Input: part model. Units: mm. Frame: model coordinates. Coordinates: 2 decimals unless noted, no trailing zeros. One line per question, with ' | ' between items. Start each with the question number.
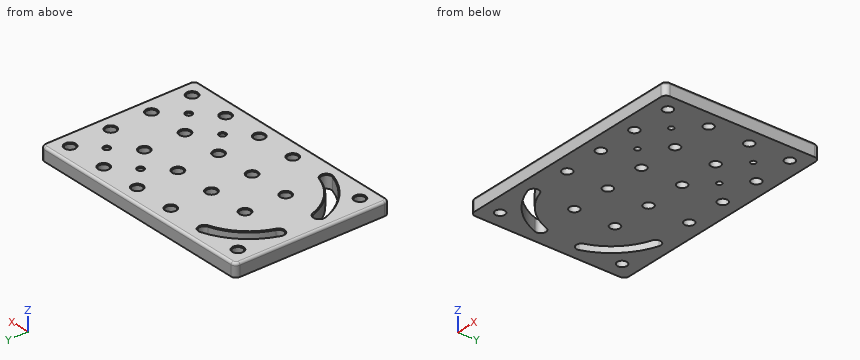
```python
from build123d import *

# Parameters (mm, degrees)
F0_W         = 145
F0_H         = 95
F0_R         = 3
F0_R_2       = 1.6
F1_DEPTH     = 8
F2_R         = 1.5
F3_SIZE      = 0.5
F4_T1_DEPTH  = 15.5
F4_T4_ANGLE  = 90
F4_T6_ANGLE  = 90
F4_T8_ANGLE  = 90
F4_T10_ANGLE = 90


# Not quite as in the source:
# - a fillet or chamfer that OpenCascade refuses, or shapes differently, is made with other operations: its cross-section is extruded or revolved along the edge and cut away or added
# - a feature names something its author has since deleted; it is built from what else it names


with BuildPart() as f1:
    # F0 (on Top) → F1 (new body)
    with BuildSketch(Plane.XY):
        with Locations((-44.7653323412, -10.0623860955)):
            Rectangle(F0_W, F0_H)
        with Locations((-107.2653323412, -47.5623860955)):
            Circle(F0_R, mode=Mode.SUBTRACT)
        with BuildLine():
            ThreePointArc((-83.2614498041, -50.5507384844), (-99.9435684207, -40.240622175), (-110.2536847301, -23.5585035585))
            ThreePointArc((-110.2536847301, -23.5585035585), (-108.2614498041, -19.5740337067), (-104.2769799523, -21.5662686326))
            ThreePointArc((-104.2769799523, -21.5662686326), (-95.4887956992, -35.7858494535), (-81.2692148782, -44.5740337067))
            ThreePointArc((-81.2692148782, -44.5740337067), (-79.2769799523, -48.5585035585), (-83.2614498041, -50.5507384844))
        make_face(mode=Mode.SUBTRACT)
        with Locations((-57.2653323412, -47.5623860955)):
            Circle(F0_R, mode=Mode.SUBTRACT)
        with Locations((-82.2653323412, -22.5623860955)):
            Circle(F0_R, mode=Mode.SUBTRACT)
        with Locations((-57.2653323412, -22.5623860955)):
            Circle(F0_R, mode=Mode.SUBTRACT)
        with Locations((-32.2653323412, -47.5623860955)):
            Circle(F0_R, mode=Mode.SUBTRACT)
        with Locations((-19.8653323412, -35.2623860955)):
            Circle(F0_R_2, mode=Mode.SUBTRACT)
        with Locations((-7.2653323412, -47.5623860955)):
            Circle(F0_R, mode=Mode.SUBTRACT)
        with Locations((17.7346676588, -47.5623860955)):
            Circle(F0_R, mode=Mode.SUBTRACT)
        with Locations((5.3346676588, -35.2623860955)):
            Circle(F0_R_2, mode=Mode.SUBTRACT)
        with Locations((-32.2653323412, -22.5623860955)):
            Circle(F0_R, mode=Mode.SUBTRACT)
        with Locations((-7.2653323412, -22.5623860955)):
            Circle(F0_R, mode=Mode.SUBTRACT)
        with Locations((17.7346676588, -22.5623860955)):
            Circle(F0_R, mode=Mode.SUBTRACT)
        with Locations((-82.2653323412, 2.4376139045)):
            Circle(F0_R, mode=Mode.SUBTRACT)
        with Locations((-57.2653323412, 2.4376139045)):
            Circle(F0_R, mode=Mode.SUBTRACT)
        with BuildLine():
            ThreePointArc((-110.2536847301, 3.4337313674), (-99.9435684207, 20.115849984), (-83.2614498041, 30.4259662933))
            ThreePointArc((-83.2614498041, 30.4259662933), (-79.2769799523, 28.4337313674), (-81.2692148782, 24.4492615156))
            ThreePointArc((-81.2692148782, 24.4492615156), (-95.4887956992, 15.6610772625), (-104.2769799523, 1.4414964415))
            ThreePointArc((-104.2769799523, 1.4414964415), (-108.2614498041, -0.5507384844), (-110.2536847301, 3.4337313674))
        make_face(mode=Mode.SUBTRACT)
        with Locations((-107.2653323412, 27.4376139045)):
            Circle(F0_R, mode=Mode.SUBTRACT)
        with Locations((-57.2653323412, 27.4376139045)):
            Circle(F0_R, mode=Mode.SUBTRACT)
        with Locations((-32.2653323412, 2.4376139045)):
            Circle(F0_R, mode=Mode.SUBTRACT)
        with Locations((-7.2653323412, 2.4376139045)):
            Circle(F0_R, mode=Mode.SUBTRACT)
        with Locations((17.7346676588, 2.4376139045)):
            Circle(F0_R, mode=Mode.SUBTRACT)
        with Locations((-19.8653323412, 15.1376139045)):
            Circle(F0_R_2, mode=Mode.SUBTRACT)
        with Locations((-32.2653323412, 27.4376139045)):
            Circle(F0_R, mode=Mode.SUBTRACT)
        with Locations((5.3346676588, 15.1376139045)):
            Circle(F0_R_2, mode=Mode.SUBTRACT)
        with Locations((-7.2653323412, 27.4376139045)):
            Circle(F0_R, mode=Mode.SUBTRACT)
        with Locations((17.7346676588, 27.4376139045)):
            Circle(F0_R, mode=Mode.SUBTRACT)
    extrude(amount=-F1_DEPTH)

    # F2
    f2_edges = [f1.edges().sort_by_distance(p)[0] for p in [
        (-117.265332, -10.062386, 0),
        (-44.765332, 37.437614, 0),
        (-44.765332, -57.562386, 0),
        (27.734668, -10.062386, 0),
    ]]
    fillet(f2_edges, radius=F2_R)

    # F3
    f3_edges = [f1.edges().sort_by_distance(p)[0] for p in [
        (-115.765332, -10.062386, 0),
        (-44.765332, 35.937614, 0),
        (-44.765332, -56.062386, 0),
        (26.234668, -10.062386, 0),
        (-110.265332, -47.562386, 0),
        (-95.488796, -35.785849, 0),
        (-79.27698, -48.558504, 0),
        (-99.943568, -40.240622, 0),
        (-108.26145, -19.574034, 0),
        (-60.265332, -47.562386, 0),
        (-85.265332, -22.562386, 0),
        (-60.265332, -22.562386, 0),
        (-35.265332, -47.562386, 0),
        (-21.465332, -35.262386, 0),
        (-10.265332, -47.562386, 0),
        (14.734668, -47.562386, 0),
        (3.734668, -35.262386, 0),
        (-35.265332, -22.562386, 0),
        (-10.265332, -22.562386, 0),
        (14.734668, -22.562386, 0),
        (-85.265332, 2.437614, 0),
        (-60.265332, 2.437614, 0),
        (-99.943568, 20.11585, 0),
        (-79.27698, 28.433731, 0),
        (-95.488796, 15.661077, 0),
        (-108.26145, -0.550738, 0),
        (-110.265332, 27.437614, 0),
        (-60.265332, 27.437614, 0),
        (-35.265332, 2.437614, 0),
        (-10.265332, 2.437614, 0),
        (14.734668, 2.437614, 0),
        (-21.465332, 15.137614, 0),
        (-35.265332, 27.437614, 0),
        (3.734668, 15.137614, 0),
        (-10.265332, 27.437614, 0),
        (14.734668, 27.437614, 0),
    ]]
    chamfer(f3_edges, length=F3_SIZE)

    # F4: fillet of radius 3 on 4 edges, made by hand

    # F4_s2 → F4_t1 (cut)
    with BuildSketch(Plane.XY.offset(-15.5)):
        with BuildLine():
            ThreePointArc((-117.2653323412, -54.5623860955), (-116.3866526848, -56.6837064391), (-114.2653323412, -57.5623860955))
            Line((-114.2653323412, -57.5623860955), (-117.2653323412, -57.5623860955))
            Line((-117.2653323412, -57.5623860955), (-117.2653323412, -54.5623860955))
        make_face()
        with BuildLine():
            ThreePointArc((24.7346676588, -57.5623860955), (26.8559880024, -56.6837064391), (27.7346676588, -54.5623860955))
            Line((27.7346676588, -54.5623860955), (27.7346676588, -57.5623860955))
            Line((27.7346676588, -57.5623860955), (24.7346676588, -57.5623860955))
        make_face()
        with BuildLine():
            ThreePointArc((24.7346676588, 37.4376139045), (26.8559880024, 36.558934248), (27.7346676588, 34.4376139045))
            Line((27.7346676588, 34.4376139045), (27.7346676588, 37.4376139045))
            Line((27.7346676588, 37.4376139045), (24.7346676588, 37.4376139045))
        make_face()
        with BuildLine():
            ThreePointArc((-117.2653323412, 34.4376139045), (-116.3866526848, 36.558934248), (-114.2653323412, 37.4376139045))
            Line((-114.2653323412, 37.4376139045), (-117.2653323412, 37.4376139045))
            Line((-117.2653323412, 37.4376139045), (-117.2653323412, 34.4376139045))
        make_face()
    extrude(amount=F4_T1_DEPTH, mode=Mode.SUBTRACT)

    # F4_s3 → F4_t4 (revolve, cut)
    with BuildSketch(Plane.YZ.offset(-114.2653323412)):
        with BuildLine():
            ThreePointArc((35.9376139045, 0), (36.9982740763, -0.4393398282), (37.4376139045, -1.5))
            Line((37.4376139045, -1.5), (37.4376139045, 0))
            Line((37.4376139045, 0), (35.9376139045, 0))
        make_face()
    revolve(axis=Axis((-114.2653323412, 34.4376139045, 0), (0, 0, 1)), revolution_arc=F4_T4_ANGLE, mode=Mode.SUBTRACT)

    # F4_s5 → F4_t6 (revolve, cut)
    with BuildSketch(Plane.XZ.offset(-34.4376139045)):
        with BuildLine():
            ThreePointArc((26.2346676588, 0), (27.2953278306, -0.4393398282), (27.7346676588, -1.5))
            Line((27.7346676588, -1.5), (27.7346676588, 0))
            Line((27.7346676588, 0), (26.2346676588, 0))
        make_face()
    revolve(axis=Axis((24.7346676588, 34.4376139045, 0), (0, 0, 1)), revolution_arc=F4_T6_ANGLE, mode=Mode.SUBTRACT)

    # F4_s7 → F4_t8 (revolve, cut)
    with BuildSketch(Plane.YZ.offset(24.7346676588)):
        with BuildLine():
            ThreePointArc((-56.0623860955, 0), (-57.1230462673, -0.4393398282), (-57.5623860955, -1.5))
            Line((-57.5623860955, -1.5), (-57.5623860955, 0))
            Line((-57.5623860955, 0), (-56.0623860955, 0))
        make_face()
    revolve(axis=Axis((24.7346676588, -54.5623860955, 0), (0, 0, 1)), revolution_arc=F4_T8_ANGLE, mode=Mode.SUBTRACT)

    # F4_s9 → F4_t10 (revolve, cut)
    with BuildSketch(Plane.XZ.offset(54.5623860955)):
        with BuildLine():
            ThreePointArc((-115.7653323412, 0), (-116.825992513, -0.4393398282), (-117.2653323412, -1.5))
            Line((-117.2653323412, -1.5), (-117.2653323412, 0))
            Line((-117.2653323412, 0), (-115.7653323412, 0))
        make_face()
    revolve(axis=Axis((-114.2653323412, -54.5623860955, 0), (0, 0, 1)), revolution_arc=F4_T10_ANGLE, mode=Mode.SUBTRACT)


solid = f1.part
```
1) Ray query, line 1 (Y direction, x = -102.5, z = -2.5); line 2 (Y direction, x = -31.5, z = -3.75); line 3 (X direction, y = -35, z = -6). Return the intervals inside material, ascending.
2) Section A-A, the plane x = -7.5. Give the number of separate pieces and of enclosed holes in the cut face, then the cut area to 3 significant figures.
3) First-contact query: P1, Ø3.5, axis at x = -57.27, y = -22.56, coming from the +Z side; P2, Ø4, axis at x = 5.33, y = -35.26, coming from the +Z side. Flat tips, straight axial feed; report the tip coordinate or a pass-through.
Answer block:
1) line 1: y = -57.56 to -37.45, -25.93 to 5.81, 17.32 to 37.44 | line 2: y = -57.56 to -50.46, -44.66 to -25.46, -19.66 to -0.46, 5.34 to 24.54, 30.34 to 37.44 | line 3: x = -117.27 to -104.4, -96.25 to -21.44, -18.29 to 3.76, 6.91 to 27.73
2) separate pieces: 5 | enclosed holes: 0 | area: 567 mm2
3) P1: passes through | P2: stops at z = -0.09
